```python
from build123d import *

# Parameters (mm, degrees)
PAD_DEPTH       = 6
SKETCH_W        = 28
SKETCH_H        = 7.4
SKETCH_W_2      = 7.4
SKETCH_H_2      = 28
PAD001_DEPTH    = 0.4
SKETCH002_R     = 1.6
POCKET_DEPTH    = 6.401
POCKET001_DEPTH = 2.5
SKETCH004_R     = 3
POCKET002_DEPTH = 1
SKETCH005_R     = 3
PAD002_DEPTH    = 0.2
CHAMFER_SIZE    = 0.4
FILLET_R        = 2


with BuildPart() as part:
    # Sketch001 → Pad (new body)
    with BuildSketch(Plane(origin=(0, -20, 0), x_dir=(1, 0, 0), z_dir=(0, 0, 1))):
        with BuildLine():
            Line((-9.5, 40.5), (9.5, 40.5))
            Line((9.5, 40.5), (9.5, -9.5))
            Line((9.5, -9.5), (-40.5, -9.5))
            Line((-40.5, -9.5), (-40.5, 9.5))
            Line((-40.5, 9.5), (-36.5, 9.5))
            ThreePointArc((-36.5, 9.5), (-32.317125, 10.922441), (-29.868569, 14.599988))
            ThreePointArc((-14.599988, 29.868569), (-25.100431, 25.100431), (-29.868569, 14.599988))
            ThreePointArc((-14.599988, 29.868569), (-10.922441, 32.317125), (-9.5, 36.5))
            Line((-9.5, 36.5), (-9.5, 40.5))
        make_face()
    extrude(amount=PAD_DEPTH)

    # Sketch → Pad001 (new body)
    with BuildSketch(Plane(origin=(0, -20, 6), x_dir=(1, 0, 0), z_dir=(0, 0, 1))):
        with Locations((-25.5, 0)):
            Rectangle(SKETCH_W, SKETCH_H)
        with Locations((0, 25.5)):
            Rectangle(SKETCH_W_2, SKETCH_H_2)
    extrude(amount=PAD001_DEPTH)

    # Sketch002 → Pocket (cut, through all)
    with BuildSketch(Plane(origin=(0, -20, 0), x_dir=(1, 0, 0), z_dir=(0, 0, -1))):
        with Locations((-33.5, 0)):
            Circle(SKETCH002_R)
        with Locations((-17.5, 0)):
            Circle(SKETCH002_R)
        with Locations((0, -17.5)):
            Circle(SKETCH002_R)
        with Locations((0, -33.5)):
            Circle(SKETCH002_R)
        with Locations((-13.5, -13.5)):
            Circle(SKETCH002_R)
    extrude(amount=-POCKET_DEPTH, mode=Mode.SUBTRACT)

    # Sketch003 → Pocket001 (cut)
    with BuildSketch(Plane(origin=(0, -20, 6), x_dir=(1, 0, 0), z_dir=(0, 0, 1))):
        Polygon((-10.598815, 11.825), (-10.598815, 15.175), (-13.5, 16.85), (-16.401185, 15.175), (-16.401185, 11.825), (-13.5, 10.15), align=None)
    extrude(amount=-POCKET001_DEPTH, mode=Mode.SUBTRACT)

    # Sketch004 → Pocket002 (cut)
    with BuildSketch(Plane(origin=(0, -20, 0), x_dir=(1, 0, 0), z_dir=(0, 0, -1))):
        with Locations((-33.5, 0)):
            Circle(SKETCH004_R)
        with Locations((-17.5, 0)):
            Circle(SKETCH004_R)
        with Locations((0, -17.5)):
            Circle(SKETCH004_R)
        with Locations((0, -33.5)):
            Circle(SKETCH004_R)
    extrude(amount=-POCKET002_DEPTH, mode=Mode.SUBTRACT)

    # Sketch005 → Pad002 (new body)
    with BuildSketch(Plane(origin=(0, -20, 1), x_dir=(1, 0, 0), z_dir=(0, 0, -1))):
        with Locations((-33.5, 0)):
            Circle(SKETCH005_R)
        with Locations((-17.5, 0)):
            Circle(SKETCH005_R)
        with Locations((0, -17.5)):
            Circle(SKETCH005_R)
        with Locations((0, -33.5)):
            Circle(SKETCH005_R)
    extrude(amount=-PAD002_DEPTH)

    # Chamfer
    chamfer_edges = [part.edges().sort_by_distance(p)[0] for p in [
        (-20.5, -20, 0),
        (-36.5, -20, 0),
        (-3, -2.5, 0),
        (-3, 13.5, 0),
    ]]
    chamfer(chamfer_edges, length=CHAMFER_SIZE)

    # Fillet
    fillet_edges = [part.edges().sort_by_distance(p)[0] for p in [
        (-32.317125, -9.077559, 0),
        (-38.5, -10.5, 0),
        (-40.5, -20, 0),
        (-40.5, -10.5, 3),
        (-25.100431, 5.100431, 0),
        (-10.922441, 12.317125, 0),
        (-9.5, 18.5, 0),
        (-9.5, 20.5, 3),
        (0, 20.5, 0),
        (9.5, 20.5, 3),
        (9.5, -4.5, 0),
        (-15.5, -29.5, 0),
        (-40.5, -29.5, 3),
        (9.5, -29.5, 3),
    ]]
    fillet(fillet_edges, radius=FILLET_R)


solid = part.part
```
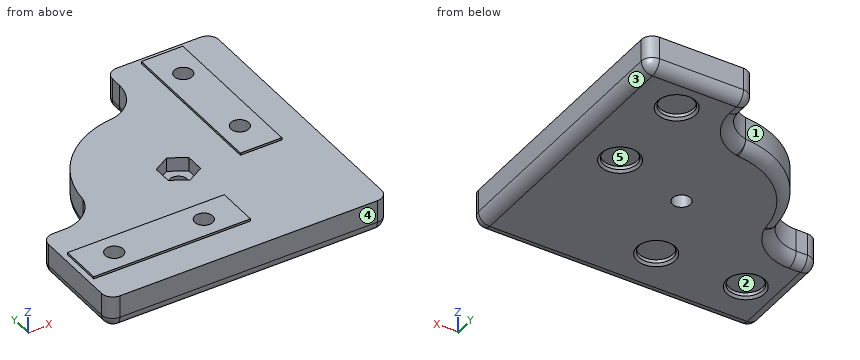
The model under review builds one solid part; all positions refer to its coordinate system, in mm. Face numbers are marked on the shaded views. A direction names the side the tool comes from. Give positions to 0.01 mm unless a question says otherwise; leave off trailing zeros. Order: outer loops, then holes, each group sorted by start corner. A loop starts at its lowest first (then second) coordinate and runs counter-clockwise, first axis right, second up. Notation, with made-up numbers: (-8, 20) - (33, 20) arc R18 ccw to (33, 45) - close; hole circle Ø2 at (82, 74.5). An arc over 180 degrees is marked (long way). Use CSV: the item, a comma, the result in double quotes. Start each with the question number.
Q1. Tool access review of the marked faces 1 and 2: name each direction out of +Z, -Z, +X, -X, +Y, -Y from which nothing blocks a thin tool from reaching the whole face with its end or side.
Q2. Clearance check with flat-ended pins moving along their axes: pin 1 Ø1 at (x, z) = (-38, 4.5) entering from +Y; pin 2 Ø1 at (x, y) = (-34, -20.5) entering from +Z; pin 3 Ø5 at (x, y) = (0, 13.5) entering from -Z. State where each tip first meets the part, or that it passes through.
Q3. To check wall thickness, follow line 1 along Y through (x, z) = (0, 3.9); line 2 along X through (y, z) = (-20, 3.4); line 3 along Y through (x, z) = (0, 0.75). State the ranges of each line that lie inside material, in increasing order. Write a range as [from, to].
Q4. We need section B-B, the plane y = -25. Write out the cut boundary in (x, z).
Q5. We need section C-C, the plane x = -5.5. Write out the cut boundary in (y, z).
Q6. The part is to be moulded in two halves that separate along X. For the marked faces 3, 4 and 5, say which applies: +X half, -X half, draft (parallel to the pull), parting line (faces both ways), or undercut.
Outcome:
1,face 1,"+Z, -Z, -X, +Y"
1,face 2,"-Z"
2,pin 1,"stops at y = -10.5"
2,pin 2,"stops at z = 1.2"
2,pin 3,"stops at z = 1"
3,line 1,"y = [-29.5, -4.1], [-0.9, 11.9], [15.1, 20.5]"
3,line 2,"x = [-40.5, -35.1], [-31.9, -19.1], [-15.9, 9.5]"
3,line 3,"y = [-29.06, -5.5], [0.5, 10.5], [16.5, 20.06]"
4,outline,"(-40.5, 2) arc R2 ccw to (-38.5, 0) - (7.5, 0) arc R2 ccw to (9.5, 2) - (9.5, 6) - (-40.5, 6) - close"
5,outline,"(-29.5, 2) arc R2 ccw to (-27.5, 0) - (18.5, 0) arc R2 ccw to (20.5, 2) - (20.5, 6) - (-29.5, 6) - close"
6,face 3,"+X half"
6,face 4,"draft"
6,face 5,"undercut"
